Read the model definition and answer for the solid it produces. Units are mm, in the model's axes. Coordinates: 2 decimals unless noted, no trailing zeros. Write each loop counter-clockwise with the first axis right and the second up, starting at its lowest first coordinate (ties: lowest second). Pieces come first, ordered by that corner, then holes. Notation, with made-up numbers: (40, 62) -> (96, 62) arc R17 cw to (96, 94) -> close; hole circle Ø5 at (24.25, 47.5). An arc over 180 degrees is marked (long way). Answer in a Markdown table with one row per item. Add a question column.
Item 1: Section C-C on y = 0.9 is taken. Write down the section's boundary in (x, z), then the cut area to 3 significant figures.
Item 2: Section B-B on z = -5 is taken. Write down the section's boundary in (x, y), then the cut area to 3 significant figures.
Item 3: Section A-A on x = 17.5 is taken. Write down the section's boundary in (y, z), then the cut area to 3 significant figures.
Item 4: Section D-D on x = 31 is taken. Write down the section's boundary in (y, z), then the cut area to 3 significant figures.
Item 5: Straight lines are drawn through the part: line 1 (X direction, y = 1.5, z = -5); line 2 (X direction, y = 1.65, z = -5.5); line 3 (Z direction, x = 31.5, y = 1.3). For each, find the intervals that lie inside material, in ascending order. Write a range as from..to.
Item 6: For a pull along X with two mould halves and no side action, classify faces 1 (the face through (-3, 1, -5)), 2 (the face through (2.8, 1, -3.4)), 3 (the face through (17.2, 2, -8.3)) as +X half, -X half, draft (parallel to the pull), parting line (faces both ways), or undercut.
Item 7: Given pin 1 Ø5 at (x, z) = (12.5, -4.5) entering from -Y, flat-ended and moving along its own axis, determine where the tip first touches the part or whether it passes through.
```python
from build123d import *

# Parameters (mm, degrees)
SKETCH1_W           = 35
SKETCH1_H           = 10
SKETCH1_R           = 3
BOSS_EXTRUDE1_DEPTH = 2
SKETCH4_R           = 2
CUT_EXTRUDE2_DEPTH  = 20
SKETCH5_W           = 10
SKETCH5_H           = 2
BOSS_EXTRUDE3_DEPTH = 3
SKETCH6_W           = 10
SKETCH6_H           = 2
BOSS_EXTRUDE4_DEPTH = 3


with BuildPart() as part:
    # Sketch1 → Boss-Extrude1 (new body)
    with BuildSketch(Plane(origin=(0, 0, 0), x_dir=(1, 0, 0), z_dir=(0, 1, 0))):
        with Locations((17.5, 5)):
            Rectangle(SKETCH1_W, SKETCH1_H)
        with Locations(Location((17.5, 5, 0), (0, 0, 270))):
            Circle(SKETCH1_R, mode=Mode.SUBTRACT)
    extrude(amount=BOSS_EXTRUDE1_DEPTH)

    # Sketch4 → Cut-Extrude2 (cut)
    with BuildSketch(Plane.XZ):
        with Locations(Location((4, -5, 0), (0, 0, 270))):
            Circle(SKETCH4_R)
        with Locations(Location((31, -5, 0), (0, 0, 270))):
            Circle(SKETCH4_R)
    extrude(amount=-CUT_EXTRUDE2_DEPTH, mode=Mode.SUBTRACT)

    # Sketch5 → Boss-Extrude3 (add)
    with BuildSketch(Plane.ZY):
        with Locations((-5, 1)):
            Rectangle(SKETCH5_W, SKETCH5_H)
    extrude(amount=BOSS_EXTRUDE3_DEPTH)

    # Sketch6 → Boss-Extrude4 (add)
    with BuildSketch(Plane(origin=(35, 0, 0), x_dir=(0, 0, -1), z_dir=(1, 0, 0))):
        with Locations((5, 1)):
            Rectangle(SKETCH6_W, SKETCH6_H)
    extrude(amount=BOSS_EXTRUDE4_DEPTH)


solid = part.part
```
Results below:
| question | item | result |
|---|---|---|
| 1 | outline | (-3, -10) -> (38, -10) -> (38, 0) -> (-3, 0) -> close; hole circle Ø4 at (4, -5); hole circle Ø6 at (17.5, -5); hole circle Ø4 at (31, -5) |
| 1 | area | 357 mm2 |
| 2 | outline | (-3, 0) -> (2, 0) -> (2, 2) -> (-3, 2) -> close; (6, 0) -> (14.5, 0) -> (14.5, 2) -> (6, 2) -> close; (20.5, 0) -> (29, 0) -> (29, 2) -> (20.5, 2) -> close; (33, 0) -> (38, 0) -> (38, 2) -> (33, 2) -> close |
| 2 | area | 54.0 mm2 |
| 3 | outline | (0, -10) -> (2, -10) -> (2, -8) -> (0, -8) -> close; (0, -2) -> (2, -2) -> (2, 0) -> (0, 0) -> close |
| 3 | area | 8.00 mm2 |
| 4 | outline | (0, -10) -> (2, -10) -> (2, -7) -> (0, -7) -> close; (0, -3) -> (2, -3) -> (2, 0) -> (0, 0) -> close |
| 4 | area | 12.0 mm2 |
| 5 | line 1 | x = -3..2, 6..14.5, 20.5..29, 33..38 |
| 5 | line 2 | x = -3..2.06, 5.94..14.54, 20.46..29.06, 32.94..38 |
| 5 | line 3 | z = -10..-6.94, -3.06..0 |
| 6 | face 1 | -X half |
| 6 | face 2 | undercut |
| 6 | face 3 | draft |
| 7 | pin 1 | stops at y = 0 |
